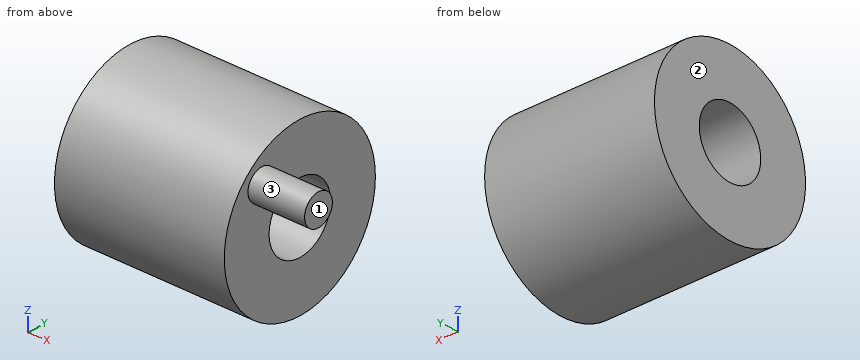
from build123d import *

# Parameters (mm, degrees)
F0_R     = 37.573612
F1_DEPTH = 76.2
F2_R     = 15.282658
F3_DEPTH = 76.2
F4_R     = 6.905206
F5_DEPTH = 25.4


with BuildPart() as f1:
    # F0 (on Right) → F1 (new body)
    with BuildSketch(Plane.YZ):
        Circle(F0_R)
    extrude(amount=F1_DEPTH)

    # F2 (on face) → F3 (cut)
    with BuildSketch(Plane.YZ.offset(76.2)):
        Circle(F2_R)
    extrude(amount=-F3_DEPTH, mode=Mode.SUBTRACT)

    # F4 (on face) → F5 (join)
    with BuildSketch(Plane.YZ.offset(76.2)):
        with Locations((-18.894237, 20.407373)):
            Circle(F4_R)
    extrude(amount=F5_DEPTH)


solid = f1.part
CAD build for the part. Positions are in the model's coordinates, mm. Face numbers are marked on the shaded views. Round coordinates to 2 decimals unless told otherwise and drop trailing zeros. Loops run counter-clockwise (first coordinate to the right, second up) from the corner with the lowest first, then second, coordinate; pieces in that order, holes last.
(1) Cut at A-A (y = 0). Give the cut face in (x, z).
(2) Wall check: line 1 along Z through (x, y) = (44, 0); line 2 along Y through (x, z) = (17, 0.5); line 3 along X through (y, z) = (-13.5, 25.5). Give the ranges that are in metal, low to high.
(3) Cut at C-C (x = 16.5). Give the cut face in (y, z), plus the area to 3 significant figures.
(4) Two-plate mould, pull along X, no slides. Class the marked faces 1, 2 and 3: +X half, -X half, draft (parallel to the pull), parting line (faces both ways), or undercut.
(5) Drop flat-ended pins along their axis: pin 1 (10 mm diameter, centred on x = 61.5, y = 8, fed in from +Z); pin 2 (5 mm diameter, centred on x = 61.5, z = 21, fed in from -Y); pin 3 (10 mm diameter, centred on x = 24.5, y = -17.5, fed in from -Z). Give the stop position or say it passes through.
(6) Cut at D-D (z = -18.5). Give the cut face in (x, y).
Findings below:
1. outline: (0, -37.57) - (76.2, -37.57) - (76.2, -15.28) - (0, -15.28) - close; (0, 15.28) - (76.2, 15.28) - (76.2, 37.57) - (0, 37.57) - close
2. line 1: z = -37.57 to -15.28, 15.28 to 37.57
2. line 2: y = -37.57 to -15.27, 15.27 to 37.57
2. line 3: x = 0 to 76.2
3. outline: circle Ø75.15 at (0, 0); hole circle Ø30.57 at (0, 0)
3. area: 3,700 mm2
4. face 1: +X half
4. face 2: -X half
4. face 3: draft
5. pin 1: stops at z = 37.45
5. pin 2: stops at y = -32.7
5. pin 3: stops at z = -35.43
6. outline: (0, -32.7) - (76.2, -32.7) - (76.2, 32.7) - (0, 32.7) - close
